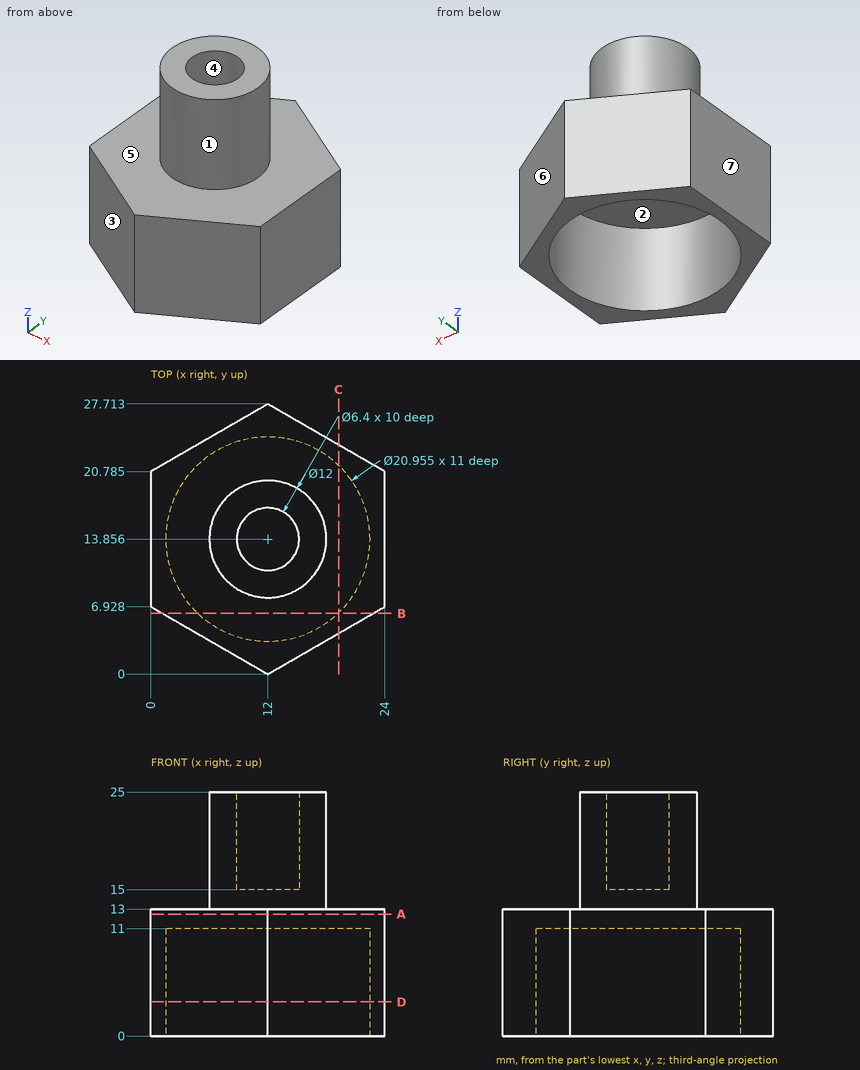
Geometry check sheet. Reference: drawing and pictorial views, mm from the part's lowest x, y, z. A direction names the side the tool comes from. Give positions to 0.01 mm unless a question says otherwise; leave off trailing zeros. Order: outer loops, then holes, each group sorted by start corner. A loop starts at its lowest first (then second) coordinate and runs counter-clockwise, first axis right, second up. Notation, with made-up numbers: M -2,4.25 L 52,4.25 A11 ccw 52,11.25 Z; hole C -2.75,76.5 d3. An arc over 180 degrees is marked long. Return JSON: item names as keys, results as strings. Group by question number.
1) Section check D-D on z = 3.5. Record the cut outline in (x, y) (1 decimal), and give its area (3 significant figures).
2) Scan lines: line 1 (Y direction, x = 12, z = 5.75) (1 decimal); line 2 (Y direction, x = 12, z = 20.25); line 3 (Z direction, x = 18, y = 20.75). Record each from-to range of solid material in increasing order.
3) Section check C-C on x = 19.25. Record the cut outline in (y, z) (1 decimal).
4) Go/stop test with flat-tipped pins: pin 1 Ø8 at (x, y) = (15, 11.5) entering from -Z; pin 2 Ø12 at (x, z) = (21.5, 12) entering from -Y; pin 3 Ø1.9 at (x, y) = (12.5, 12.5) entering from +Z. Record where each tip stops, or that it passes through.
5) Section check B-B on y = 6.25. Record the cut outline in (x, z) (1 decimal), and give its area (3 significant figures).
6) Mould release check, pull along X, two halves, no side actions. Record for the marked faces 4, 5, 6 and 7: pulls with the +X half, pulls with the -X half, needs draft (parallel to the pull), parting line crosses it, or undercut.
7) Access from +Z, -Z, +X, -X, +Y, -Y to the whole of each face (thin tool, end or side, straight path). Record for the marked faces 1, 2 and 3.
8) Section check A-A on z = 12.5. Record the cut outline in (x, y) (1 decimal).
Answer block:
{
 "1": {"outline": "M 0,6.9 L 12,0 L 24,6.9 L 24,20.8 L 12,27.7 L 0,20.8 Z; hole C 12,13.9 d21", "area": "154 mm^2"},
 "2": {"line 1": "y = 0 to 3.4, 24.3 to 27.7", "line 2": "y = 7.86 to 10.66, 17.06 to 19.86", "line 3": "z = 11 to 13"},
 "3": {"outline": "M 4.2,0 L 6.3,0 L 6.3,11 L 21.4,11 L 21.4,0 L 23.5,0 L 23.5,13 L 4.2,13 Z"},
 "4": {"pin 1": "stops at z = 11", "pin 2": "stops at y = 2.02", "pin 3": "stops at z = 15"},
 "5": {"outline": "M 1.2,0 L 4.8,0 L 4.8,11 L 19.2,11 L 19.2,0 L 22.8,0 L 22.8,13 L 1.2,13 Z", "area": "123 mm^2"},
 "6": {"face 4": "undercut", "face 5": "needs draft", "face 6": "pulls with the +X half", "face 7": "pulls with the -X half"},
 "7": {"face 1": "+Z", "face 2": "-Z", "face 3": "+Z, -Z, -X, -Y"},
 "8": {"outline": "M 0,6.9 L 12,0 L 24,6.9 L 24,20.8 L 12,27.7 L 0,20.8 Z"}
}
